Build history of the part. All positions in model axes, mm. A direction names the side the tool comes from. Round coordinates to 2 decimals unless told otherwise and drop trailing zeros. Write each loop counter-clockwise with the first axis right and the second up, starting at its lowest first coordinate (ties: lowest second). Pieces come first, ordered by that corner, then holes. Notation, with made-up numbers: M 73,84 L 118,84 A24 cw 118,112 Z; hole C 14.5,-29.5 d1. An arc over 180 degrees is marked long. Use a Markdown table: item, result.
from build123d import *

# Parameters (mm, degrees)
SKETCH_1_R          = 7.5
EXTRUDE_1_DEPTH     = 8
FILLET_1_R          = 5
SKETCH_2_W          = 5
SKETCH_2_H          = 6
CUT_EXTRUDE_1_DEPTH = 8
SKETCH_3_W          = 10
SKETCH_3_H          = 8
EXTRUDE_2_DEPTH     = 5
SKETCH_4_W          = 8
SKETCH_4_H          = 8
CUT_EXTRUDE_2_DEPTH = 60.438258903


with BuildPart() as part:
    # 草图1 → 凸台-拉伸1 (new body)
    with BuildSketch(Plane.XY):
        Polygon((2.970014974, 11), (22.908786289, 30.938771315), (22.908786289, 37.998771315), (45, 37.998771315), (45, 0), (2.007639675, 0), align=None)
        with Locations((22.5, 13)):
            Circle(SKETCH_1_R, mode=Mode.SUBTRACT)
    extrude(amount=EXTRUDE_1_DEPTH)

    # 圆角1
    fillet_1_edges = [part.edges().sort_by_distance(p)[0] for p in [
        (2.970014974, 11, 4),
        (22.908786289, 30.938771315, 4),
    ]]
    fillet(fillet_1_edges, radius=FILLET_1_R)

    # 草图2 → 切除-拉伸1 (cut)
    with BuildSketch(Plane.XY.offset(8)):
        with Locations((32, 34.998771315)):
            Rectangle(SKETCH_2_W, SKETCH_2_H)
    extrude(amount=-CUT_EXTRUDE_1_DEPTH, mode=Mode.SUBTRACT)

    # 草图3 → 凸台-拉伸2 (add)
    with BuildSketch(Plane.XZ):
        with Locations((40, 4)):
            Rectangle(SKETCH_3_W, SKETCH_3_H)
        with Locations((5, 4)):
            Rectangle(SKETCH_3_W, SKETCH_3_H)
    extrude(amount=EXTRUDE_2_DEPTH)

    # 草图4 → 切除-拉伸2 (cut, through all)
    with BuildSketch(Plane.XY.offset(8)):
        with Locations((41, 12)):
            Rectangle(SKETCH_4_W, SKETCH_4_H)
        with Locations((41, 28)):
            Rectangle(SKETCH_4_W, SKETCH_4_H)
    extrude(amount=-CUT_EXTRUDE_2_DEPTH, mode=Mode.SUBTRACT)


solid = part.part
Q1. Cut at B-B on z = 3.5. Give the cut face in (x, y), and give its area (3 significant figures).
Response values:
| item | result |
|---|---|
| outline | M 0,-5 L 10,-5 L 10,0 L 35,0 L 35,-5 L 45,-5 L 45,8 L 37,8 L 37,16 L 45,16 L 45,24 L 37,24 L 37,32 L 45,32 L 45,38 L 34.5,38 L 34.5,32 L 29.5,32 L 29.5,38 L 22.91,38 L 22.91,33.01 A5 cw 21.44,29.47 L 4.26,12.29 A5 ccw 2.81,9.19 L 2.01,0 L 0,0 Z; hole C 22.5,13 d15 |
| area | 1,030 mm2 |
Q2. Drill centre lines: L1, parallel to X at y = 33, z = 7; L2, parallel to Y at x = 21.5, z = 1.25; L3, parallel to Y at x = 22.5, z = 2.25. Where is each one in solid material? Low to high.
Response values:
| item | result |
|---|---|
| L1 | x = 22.91 to 29.5, 34.5 to 45 |
| L2 | y = 0 to 5.57, 20.43 to 29.53 |
| L3 | y = 0 to 5.5, 20.5 to 31.03 |
Q3. Cut at A-A on y = 34. Give the cut face in (x, z), and give its area (3 significant figures).
Response values:
| item | result |
|---|---|
| outline | M 22.91,0 L 29.5,0 L 29.5,8 L 22.91,8 Z; M 34.5,0 L 45,0 L 45,8 L 34.5,8 Z |
| area | 137 mm2 |
Q4. Drop flat-ended pins along their axis: P1, Ø4, axis at x = 28.5, z = 4, coming from the -Y side; P2, Ø1.5, axis at y = 36, z = 5, coming from the -X side; P3, Ø1, axis at y = 12.5, z = 6.5, coming from the +X side. Give the stop position or say it passes through.
Response values:
| item | result |
|---|---|
| P1 | stops at y = 0 |
| P2 | stops at x = 22.91 |
| P3 | stops at x = 37 |
Q5. Cut at C-C on x = 16.5. Give the cut face in (y, z), and give its area (3 significant figures).
Response values:
| item | result |
|---|---|
| outline | M 0,0 L 8.5,0 L 8.5,8 L 0,8 Z; M 17.5,0 L 24.53,0 L 24.53,8 L 17.5,8 Z |
| area | 124 mm2 |
Q6. Two-plate mould, pull along X, no slides. Class faces 5 (the cylindrical face through (3.271, 10.887, 4.056)), 6 (the flat face through (29.5, 35, 4)), 7 (the flat face through (41, 16, 4)): +X half, -X half, draft (parallel to the pull), parting line (faces both ways), or undercut.
Response values:
| item | result |
|---|---|
| face 5 | -X half |
| face 6 | undercut |
| face 7 | draft |
Q7. Cut at D-D on y = 26. Give the cut face in (x, z), and give its area (3 significant figures).
Response values:
| item | result |
|---|---|
| outline | M 17.97,0 L 37,0 L 37,8 L 17.97,8 Z |
| area | 152 mm2 |
Q8. Which spindle directions (+Z, -Z, +X, -X, +Y, -Y) get a long thin tool onto all of the face, cutting with end or side? Do faces 1 (the flat face through (5, -5, 4)), 2 (the flat face through (1, 0, 4)), 3 (the flat face through (41, 32, 4)), 4 (the flat face through (32, 31.999, 4)). Say none if no direction does.
Response values:
| item | result |
|---|---|
| face 1 | +Z, -Z, +X, -X, -Y |
| face 2 | +Z, -Z, -X, +Y |
| face 3 | +Z, -Z, +X |
| face 4 | +Z, -Z, +Y |
